Check sheet for the modelled part. Datum: model origin and axes. Units: mm. A direction names the side the tool comes from. Round coordinates to 2 decimals unless told otherwise and drop trailing zeros. Order: outer loops, then holes, each group sorted by start corner. A loop starts at its lowest first (then second) coordinate and runs counter-clockwise, first axis right, second up. Notation, with made-up numbers: (59.5, 41.25) -> (92.5, 41.25) arc R21 cw to (92.5, 66.25) -> close; hole circle Ø4 at (-35, 48.25). An arc over 180 degrees is marked (long way). Use CSV: the item, a comma, the result in double quotes.
```python
from build123d import *

# Parameters (mm, degrees)
SKETCH1_W                = 19.05
SKETCH1_H                = 19.05
BOSS_EXTRUDE1_DEPTH      = 15.24
SKETCH2_W                = 19.05
SKETCH2_H                = 2.54
BOSS_EXTRUDE2_DEPTH      = 3.8608
SKETCH3_W                = 5.715
SKETCH3_H                = 0.317516884
BOSS_EXTRUDE3_DEPTH      = 3.8608
SKETCH4_R                = 0.254
CUT_EXTRUDE1_DEPTH       = 3.8608
CUT_EXTRUDE2_DEPTH       = 16.51
BOSS_EXTRUDE4_DEPTH      = 10.16
BOSS_EXTRUDE4_DEPTH_BACK = 29.21
SKETCH6_W                = 15.312192665
SKETCH6_H                = 16.51
SKETCH7_OUTSIDE_W        = 36.524
SKETCH7_OUTSIDE_H        = 49.122
SKETCH7_OUTSIDE_R        = 7.112
CUT_EXTRUDE3_DEPTH       = 10.16
SKETCH8_OUTSIDE_W        = 36.524
SKETCH8_OUTSIDE_H        = 49.122
SKETCH8_OUTSIDE_R        = 7.112
CUT_EXTRUDE4_DEPTH       = 10.16
SKETCH9_W                = 19.05
SKETCH9_H                = 15.312192665
SKETCH9_R                = 5.588
CUT_EXTRUDE6_DEPTH       = 10.16
SKETCH10_R               = 5.238445082
BOSS_EXTRUDE5_DEPTH      = 20.32
BOSS_EXTRUDE6_DEPTH      = 2.54
BOSS_EXTRUDE6_DEPTH_BACK = 17.78
SKETCH11_W               = 19.05
SKETCH11_H               = 6.35
FILLET1_R                = 1.524
FILLET2_R                = 1.016
FILLET3_R                = 1.016
FILLET5_R                = 0.762
FILLET6_R                = 0.254
SKETCH12_R               = 3.81
CUT_EXTRUDE7_DEPTH       = 58.807833199


with BuildPart() as part:
    # Sketch1 → Boss-Extrude1 (new body)
    with BuildSketch(Plane.XY):
        with Locations((9.525, 9.525)):
            Rectangle(SKETCH1_W, SKETCH1_H)
    extrude(amount=BOSS_EXTRUDE1_DEPTH)

    # Sketch2 → Boss-Extrude2 (add)
    with BuildSketch(Plane.XY.offset(15.24)):
        with Locations((9.525, 1.27)):
            Rectangle(SKETCH2_W, SKETCH2_H)
    extrude(amount=BOSS_EXTRUDE2_DEPTH)

    # Sketch3 → Boss-Extrude3 (add)
    with BuildSketch(Plane.XY.offset(19.1008)):
        with Locations((14.2875, 1.428758442)):
            Rectangle(SKETCH3_W, SKETCH3_H)
        with Locations((4.7625, 1.428758442)):
            Rectangle(SKETCH3_W, SKETCH3_H)
    extrude(amount=BOSS_EXTRUDE3_DEPTH)

    # Sketch4 → Cut-Extrude1 (cut)
    with BuildSketch(Plane(origin=(0, 1.587516884, 0), x_dir=(1, 0, 0), z_dir=(0, 1, 0))):
        with Locations(Location((4.7625, -21.0312, 0), (0, 0, 180))):
            Circle(SKETCH4_R)
        with Locations(Location((14.2875, -21.0312, 0), (0, 0, 180))):
            Circle(SKETCH4_R)
    extrude(amount=-CUT_EXTRUDE1_DEPTH, mode=Mode.SUBTRACT)

    # Sketch5 → Cut-Extrude2 (cut)
    with BuildSketch(Plane(origin=(0, 19.05, 0), x_dir=(1, 0, 0), z_dir=(0, 1, 0))):
        with BuildLine():
            ThreePointArc((15.673821391, -10.861568969), (13.115527413, -13.571796937), (9.525, -14.57095489))
            Line((9.525, -14.57095489), (9.525, -15.24))
            Line((9.525, -15.24), (15.673821391, -15.24))
            Line((15.673821391, -15.24), (15.673821391, -10.861568969))
        make_face()
        with BuildLine():
            ThreePointArc((9.525, -14.57095489), (5.934472587, -13.571796937), (3.376178609, -10.861568969))
            Line((3.376178609, -10.861568969), (3.376178609, -15.24))
            Line((3.376178609, -15.24), (9.525, -15.24))
            Line((9.525, -15.24), (9.525, -14.57095489))
        make_face()
        with BuildLine():
            Line((9.525, 0), (3.376178609, 0))
            Line((3.376178609, 0), (3.376178609, -4.378431031))
            ThreePointArc((3.376178609, -4.378431031), (5.934472587, -1.668203063), (9.525, -0.66904511))
            Line((9.525, -0.66904511), (9.525, 0))
        make_face()
        with BuildLine():
            Line((15.673821391, 0), (9.525, 0))
            Line((9.525, 0), (9.525, -0.66904511))
            ThreePointArc((9.525, -0.66904511), (13.115527413, -1.668203063), (15.673821391, -4.378431031))
            Line((15.673821391, -4.378431031), (15.673821391, 0))
        make_face()
    extrude(amount=-CUT_EXTRUDE2_DEPTH, mode=Mode.SUBTRACT)

    # Sketch6 → Boss-Extrude4 (add, two sides: drawn at the far end of the back side and taken through both)
    with BuildSketch(Plane.ZY.offset(-BOSS_EXTRUDE4_DEPTH_BACK)):
        with Locations((7.656096333, 27.305)):
            Rectangle(SKETCH6_W, SKETCH6_H)
    extrude(amount=BOSS_EXTRUDE4_DEPTH + BOSS_EXTRUDE4_DEPTH_BACK)

    # Sketch7 outside → Cut-Extrude3 (cut)
    with BuildSketch(Plane.ZY.offset(10.16)):
        with Locations((11.481, 17.78)):
            Rectangle(SKETCH7_OUTSIDE_W, SKETCH7_OUTSIDE_H)
        with Locations((7.656096333, 27.94)):
            Circle(SKETCH7_OUTSIDE_R, mode=Mode.SUBTRACT)
    extrude(amount=-CUT_EXTRUDE3_DEPTH, mode=Mode.SUBTRACT)

    # Sketch8 outside → Cut-Extrude4 (cut)
    with BuildSketch(Plane(origin=(29.21, 0, 0), x_dir=(0, 0, -1), z_dir=(1, 0, 0))):
        with Locations((-11.481, 17.78)):
            Rectangle(SKETCH8_OUTSIDE_W, SKETCH8_OUTSIDE_H)
        with Locations(Location((-7.656096333, 27.94, 0), (0, 0, 180))):
            Circle(SKETCH8_OUTSIDE_R, mode=Mode.SUBTRACT)
    extrude(amount=-CUT_EXTRUDE4_DEPTH, mode=Mode.SUBTRACT)

    # Sketch9 → Cut-Extrude6 (cut)
    with BuildSketch(Plane(origin=(0, 35.56, 0), x_dir=(1, 0, 0), z_dir=(0, 1, 0))):
        with Locations((9.525, -7.656096333)):
            Rectangle(SKETCH9_W, SKETCH9_H)
        with Locations(Location((9.525, -7.656096333, 0), (0, 0, 270))):
            Circle(SKETCH9_R, mode=Mode.SUBTRACT)
    extrude(amount=-CUT_EXTRUDE6_DEPTH, mode=Mode.SUBTRACT)

    # Sketch10 → Boss-Extrude5 (add)
    with BuildSketch(Plane(origin=(0, 0, 0), x_dir=(0, 0, -1), z_dir=(1, 0, 0))):
        with Locations((-7.656096333, 27.94)):
            Circle(SKETCH10_R)
    extrude(amount=BOSS_EXTRUDE5_DEPTH)

    # Sketch11 → Boss-Extrude6 (add, two sides: drawn at the far end of the back side and taken through both)
    with BuildSketch(Plane.XY.offset(15.312192665).offset(-BOSS_EXTRUDE6_DEPTH_BACK)):
        with Locations((9.525, 22.225)):
            Rectangle(SKETCH11_W, SKETCH11_H)
        Polygon((0, 19.05), (0, 25.4), (-2.54, 25.4), (-2.54, 18.996030985), (0, 18.996030985), align=None)
        Polygon((21.59, 25.4), (19.05, 25.4), (19.05, 19.05), (0, 19.05), (0, 18.996030985), (21.59, 18.996030985), align=None)
    extrude(amount=BOSS_EXTRUDE6_DEPTH + BOSS_EXTRUDE6_DEPTH_BACK)

    # Fillet1
    fillet1_edges = [part.edges().sort_by_distance(p)[0] for p in [
        (-2.54, 25.4, 16.075625494),
        (9.525, 25.4, -2.467807335),
        (-2.54, 25.4, -0.727336496),
        (-2.54, 22.198015493, -2.467807335),
        (21.59, 25.4, 16.075625494),
        (21.59, 22.198015493, 17.852192665),
        (21.59, 25.4, -0.727336496),
        (21.59, 22.198015493, -2.467807335),
        (9.525, 25.4, 17.852192665),
        (-2.54, 22.198015493, 17.852192665),
    ]]
    fillet(fillet1_edges, radius=FILLET1_R)

    # Fillet2
    fillet2_edges = [part.edges().sort_by_distance(p)[0] for p in [
        (9.525, 35.56, 2.068096333),
    ]]
    fillet(fillet2_edges, radius=FILLET2_R)

    # Fillet3
    fillet3_edges = [part.edges().sort_by_distance(p)[0] for p in [
        (-10.16, 27.94, 0.544096333),
        (29.21, 27.94, 0.544096333),
    ]]
    fillet(fillet3_edges, radius=FILLET3_R)

    # Fillet5
    # the kernel refuses this fillet: 0.762 mm, written as the material it takes off along each edge
    with BuildSketch(Plane(origin=(17.145, 3.492516884, 22.9616), x_dir=(0, 0, -1), z_dir=(0, -1, 0)), Plane(origin=(1.905, -0.635, 22.9616), x_dir=(0, 0, -1), z_dir=(0, 1, 0))) as fillet5_piece_1:
        with BuildLine():
            CenterArc((FILLET5_R, -FILLET5_R), FILLET5_R, 90, 90)
            Line((0, -FILLET5_R), (-FILLET5_R * 0.02, -FILLET5_R))
            Line((-FILLET5_R * 0.02, -FILLET5_R), (-FILLET5_R * 0.02, FILLET5_R * 0.02))
            Line((-FILLET5_R * 0.02, FILLET5_R * 0.02), (FILLET5_R, FILLET5_R * 0.02))
            Line((FILLET5_R, FILLET5_R * 0.02), (FILLET5_R, 0))
        make_face()
    fillet5_piece_1_solid = extrude(amount=4.127516884, mode=Mode.PRIVATE)
    with BuildSketch(Plane(origin=(9.882666084, 1.587516884, 22.9616), x_dir=(0, 0, -1), z_dir=(1, 0, 0)), Plane(origin=(0.357666084, 1.587516884, 22.9616), x_dir=(0, 0, -1), z_dir=(1, 0, 0))) as fillet5_piece_2:
        with BuildLine():
            CenterArc((0.618933566, -0.762), FILLET5_R, 90, 54.316228291)
            Line((0, -0.317516884), (-0.012378671, -0.308627222))
            ThreePointArc((-0.012378671, -0.308627222), (-0.01524, -0.158758442), (-0.01524, 0))
            Line((-0.01524, 0), (0, 0.01524))
            Line((0, 0.01524), (0.618933566, 0.01524))
            Line((0.618933566, 0.01524), (0.618933566, 0))
        make_face()
    fillet5_piece_2_solid = extrude(amount=8.809667832, mode=Mode.PRIVATE)
    add([fillet5_piece_1_solid, fillet5_piece_2_solid], mode=Mode.SUBTRACT)

    # Fillet6
    fillet6_edges = [part.edges().sort_by_distance(p)[0] for p in [
        (0, 2.54, 17.1704),
        (19.05, 2.54, 17.1704),
        (9.525, 2.54, 19.1008),
        (9.525, 2.54, 0),
    ]]
    fillet(fillet6_edges, radius=FILLET6_R)

    # Sketch12 → Cut-Extrude7 (cut, through all)
    with BuildSketch(Plane.ZY.offset(10.16)):
        with Locations((7.656096333, 27.94)):
            Circle(SKETCH12_R)
    extrude(amount=-CUT_EXTRUDE7_DEPTH, mode=Mode.SUBTRACT)


solid = part.part
```
Q1. Mould release check, pull along Y, two halves, no side actions. Record for faces 1 (the face through (9, 21, -2.468)), 2 (the face through (4.7, 1.27, 20.6)), 3 (the face through (21.132, 24.965, 15.245)), 4 (the face through (-2.105, 24.942, 0.15)): pulls with the +Y half, pulls with the -Y half, needs draft (parallel to the pull), parting line crosses it, or undercut.
Result sheet:
face 1,"needs draft"
face 2,"pulls with the -Y half"
face 3,"undercut"
face 4,"undercut"
Q2. Sectioned sample at A-A, the plane y = 27.94. Enter the section's corners in (x, z) (3 decimals), then the cut area to 3 significant figures.
Result sheet:
outline,"(-10.16, 1.56) arc R1.016 ccw to (-9.144, 0.544) -> (0, 0.544) -> (0, 2.418) -> (7.58, 2.418) arc R5.588 ccw to (11.47, 2.418) -> (19.05, 2.418) -> (19.05, 0.544) -> (28.194, 0.544) arc R1.016 ccw to (29.21, 1.56) -> (29.21, 3.846) -> (-10.16, 3.846) -> close; (-10.16, 11.466) -> (29.21, 11.466) -> (29.21, 13.752) arc R1.016 ccw to (28.194, 14.768) -> (19.05, 14.768) -> (19.05, 12.895) -> (11.47, 12.895) arc R5.588 ccw to (7.58, 12.895) -> (0, 12.895) -> (0, 14.768) -> (-9.144, 14.768) arc R1.016 ccw to (-10.16, 13.752) -> close"
area,"190 mm^2"
Q3. Go/stop test with flat-tipped pins: pin 1 (2 mm diameter, centred on x = 0.5, y = 5.5, fed in from -Z); pin 2 (5 mm diameter, centred on y = 12.5, z = 14, fed in from +X); pin 3 (1 mm diameter, centred on x = 1.5, y = 13, fed in from +Z); pin 4 (3 mm diameter, centred on y = 31, z = 1, fed in from +X). Record where each tip stops, or that it passes through.
Result sheet:
pin 1,"stops at z = 0"
pin 2,"stops at x = 19.05"
pin 3,"stops at z = 15.24"
pin 4,"stops at x = 29.21"
Q4. Access from +Z, -Z, +X, -X, +Y, -Y to the whole of each face (thin tool, end or side, straight path). Record for faces 5 (the face through (2.895, 33.176, 7.504)), 6 (the face through (19.05, 10, 8)), 7 (the face through (-4.64, 34.99, 6.73)).
Result sheet:
face 5,"none"
face 6,"+Z, -Z, +X, -Y"
face 7,"-X"
Q5. Sectioned sample at C-C, the plane x = 21. Enter the section's corners in (y, z), then the cut area to 3 significant figures.
Result sheet:
outline,"(19, -2.15) -> (23.88, -2.15) arc R1.2 ccw to (25.08, -0.94) -> (25.08, 1.14) arc R7.11 ccw (long way) to (25.08, 14.17) -> (25.08, 16.33) arc R1.2 ccw to (23.88, 17.53) -> (19, 17.53) -> close; hole circle Ø7.62 at (27.94, 7.66)"
area,"193 mm^2"
Q6. Scan lines: L1, parallel to Z at x = 9.5, y = 33; L2, parallel to Y at x = 16.5, z = 14; L3, parallel to Y at x = 15, z = 1.5. Record each from-to range of solid material in increasing order.
Result sheet:
L1,"z = 2.07 to 13.24"
L2,"y = 0 to 25.4"
L3,"y = 0 to 2.54, 19 to 25.4"
Q7. Sectioned sample at B-B, the plane x = 26. Enter the section's corners in (y, z).
Result sheet:
outline,"circle Ø14.22 at (27.94, 7.66); hole circle Ø7.62 at (27.94, 7.66)"
